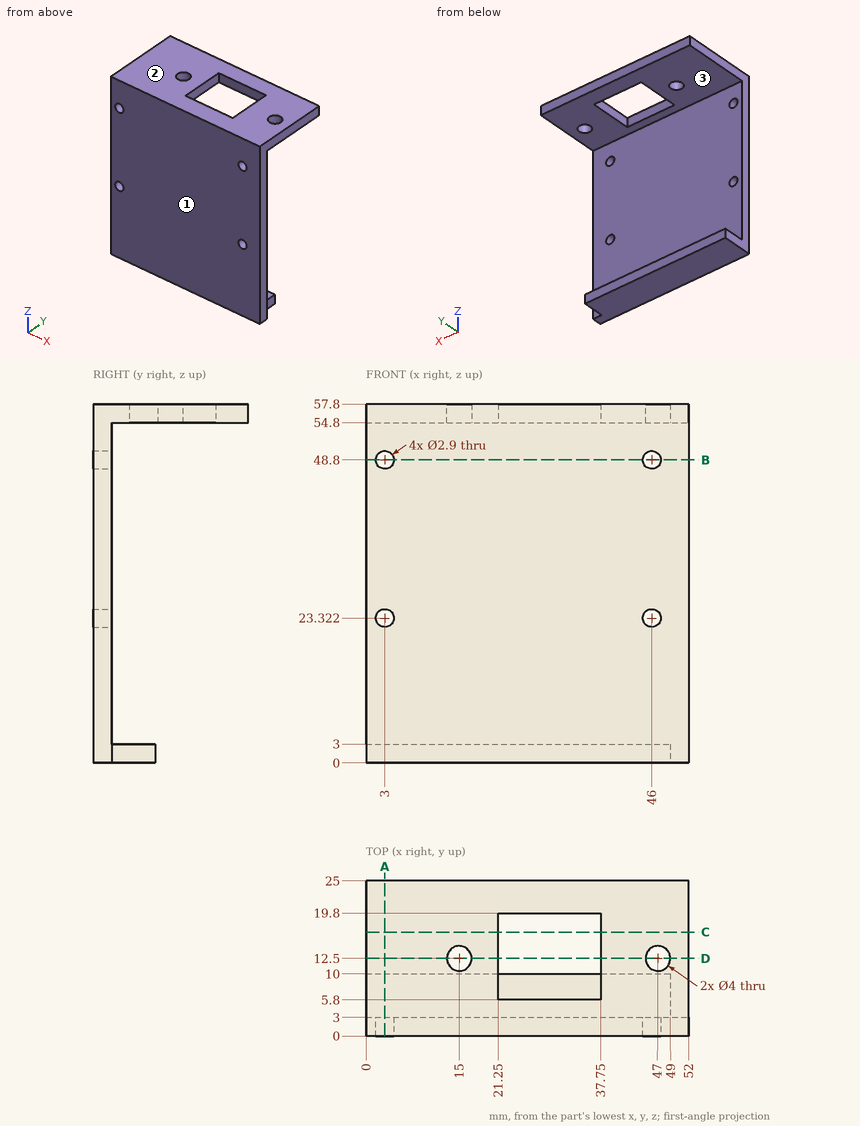
The drawing under review shows one solid part. Ordinate dimensions are in mm from its lowest x, y, z. Give positions to 0.01 mm unless a question says otherwise; leave off trailing zeros. Write each loop counter-clockwise with the first axis right and the second up, starting at its lowest first coordinate (ties: lowest second). Pieces come first, ordered by that corner, then holes. Notation, with made-up numbers: M 83.5,60.5 L 90.5,60.5 A7 cw 90.5,71.5 Z; hole C -22,51 d11. An arc over 180 degrees is marked long. Write each question's results on one line, items separated by ' | '. Start each with the question number.
1. Mouldability with a two-part tool opening along Z and no side actions: class the marked faces 1, 2 and 3 as released by +Z, released by -Z, zero draft, split by the parting line, or undercut.
2. Insertion check: pin 1 Ø3 at (x, y) = (47, 12.5) entering from -Z; pin 2 Ø4 at (x, z) = (3, 48.8) entering from +Y; pin 3 Ø0.9 at (y, z) = (7.5, 1) entering from +X; pin 4 Ø1.5 at (x, y) = (38, 14.5) entering from -Z. Each pin has a flat end and moves straight along its axis. Give the tip position at first contact, or say it passes through.
3. We need section B-B (z = 48.8). Write out the cut boundary in (x, y), and give its area (3 significant figures).
4. We need section D-D (y = 12.5). Write out the cut boundary in (x, z).
5. We need section A-A (x = 3). Write out the cut boundary in (y, z).
6. We need section C-C (y = 16.75). Write out the cut boundary in (x, z), and give its area (4 significant figures).
7. For probe 1 along Z at (x, y) = (46, 2.2); probe 2 along X at (y, z) = (1.2, 48.8); probe 3 along Z at (x, y) = (13, 9.75), list the stretches that pass through material, from the lowest coordinate up. Write a range as [from, to].
Results found:
1) face 1: zero draft | face 2: released by +Z | face 3: undercut
2) pin 1: passes through | pin 2: stops at y = 3 | pin 3: stops at x = 49 | pin 4: stops at z = 54.8
3) outline: M 0,0 L 1.55,0 L 1.55,3 L 0,3 Z; M 4.45,0 L 44.55,0 L 44.55,3 L 4.45,3 Z; M 47.45,0 L 52,0 L 52,3 L 47.45,3 Z | area: 139 mm^2
4) outline: M 0,54.8 L 13,54.8 L 13,57.8 L 0,57.8 Z; M 17,54.8 L 21.25,54.8 L 21.25,57.8 L 17,57.8 Z; M 37.75,54.8 L 45,54.8 L 45,57.8 L 37.75,57.8 Z; M 49,54.8 L 52,54.8 L 52,57.8 L 49,57.8 Z
5) outline: M 0,0 L 10,0 L 10,3 L 3,3 L 3,21.87 L 0,21.87 Z; M 0,24.77 L 3,24.77 L 3,47.35 L 0,47.35 Z; M 0,50.25 L 3,50.25 L 3,54.8 L 25,54.8 L 25,57.8 L 0,57.8 Z
6) outline: M 0,54.8 L 21.25,54.8 L 21.25,57.8 L 0,57.8 Z; M 37.75,54.8 L 52,54.8 L 52,57.8 L 37.75,57.8 Z | area: 106.5 mm^2
7) probe 1: z = [0, 21.87], [24.77, 47.35], [50.25, 57.8] | probe 2: x = [0, 1.55], [4.45, 44.55], [47.45, 52] | probe 3: z = [0, 3], [54.8, 57.8]
